```python
from build123d import *

# Parameters (mm, degrees)
SKETCH1_R           = 21
SKETCH1_R_2         = 6
BOSS_EXTRUDE1_DEPTH = 6
SKETCH2_R           = 10.5
SKETCH2_R_2         = 6
BOSS_EXTRUDE2_DEPTH = 24
SKETCH3_R           = 9.75
SKETCH3_R_2         = 6.75
CUT_EXTRUDE1_DEPTH  = 1
CUT_EXTRUDE2_START  = -7
SKETCH4_R           = 3.4
CUT_EXTRUDE2_DEPTH  = 32
CIRPATTERN1_COUNT   = 4


with BuildPart() as part:
    # Sketch1 → Boss-Extrude1 (new body)
    with BuildSketch(Plane(origin=(0, 0, 0), x_dir=(1, 0, 0), z_dir=(0, 1, 0))):
        Circle(SKETCH1_R)
        Circle(SKETCH1_R_2, mode=Mode.SUBTRACT)
    extrude(amount=BOSS_EXTRUDE1_DEPTH)

    # Sketch2 → Boss-Extrude2 (add)
    with BuildSketch(Plane(origin=(0, 6, 0), x_dir=(1, 0, 0), z_dir=(0, 1, 0))):
        Circle(SKETCH2_R)
        Circle(SKETCH2_R_2, mode=Mode.SUBTRACT)
    extrude(amount=BOSS_EXTRUDE2_DEPTH)

    # Sketch3 → Cut-Extrude1 (cut)
    with BuildSketch(Plane(origin=(0, 30, 0), x_dir=(1, 0, 0), z_dir=(0, 1, 0))):
        Circle(SKETCH3_R)
        Circle(SKETCH3_R_2, mode=Mode.SUBTRACT)
    extrude(amount=-CUT_EXTRUDE1_DEPTH, mode=Mode.SUBTRACT)

    # Sketch4 → Cut-Extrude2 (cut)
    with BuildSketch(Plane(origin=(0, 6, 0), x_dir=(1, 0, 0), z_dir=(0, 1, 0)).offset(CUT_EXTRUDE2_START)):
        with Locations((16, 0)):
            Circle(SKETCH4_R)
    cut_extrude2 = extrude(amount=CUT_EXTRUDE2_DEPTH, mode=Mode.SUBTRACT)

    # CirPattern1: Cut-Extrude2 ×4 about axis
    cirpattern1_axis = Axis((0, 0, 0), (0, 1, 0))
    for i in range(1, CIRPATTERN1_COUNT):
        add(cut_extrude2.rotate(cirpattern1_axis, i * 360 / CIRPATTERN1_COUNT), mode=Mode.SUBTRACT)


solid = part.part
```
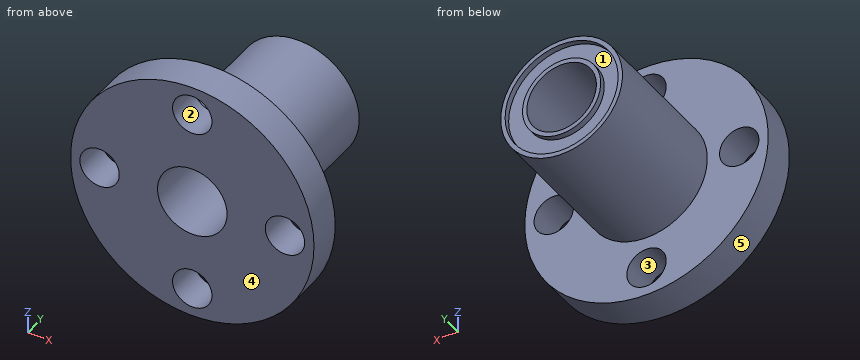
The model under review builds one solid part; all positions refer to its coordinate system, in mm. Face numbers are marked on the shaded views. A direction names the side the tool comes from. Round coordinates to 2 decimals unless told otherwise and drop trailing zeros. Loops run counter-clockwise (first coordinate to the right, second up) from the corner with the lowest first, then second, coordinate; pieces in that order, holes last.
1) Consider section C-C on z = 16. State the section outline as (x, y) points.
Values follow:
outline: (-13.6, 0) - (-3.4, 0) - (-3.4, 6) - (-13.6, 6) - close; (3.4, 0) - (13.6, 0) - (13.6, 6) - (3.4, 6) - close
2) Wall thickness on line 1 along X through (y, z) = (29.35, 0); line 2 along X through (y, z) = (18.25, 0); line 3 along Y through (x, z) = (16, -6): over which ranges is each line inside the solid? List them lowest first.
Values follow:
line 1: x = -10.5 to -9.75, -6.75 to -6, 6 to 6.75, 9.75 to 10.5
line 2: x = -10.5 to -6, 6 to 10.5
line 3: y = 0 to 6
3) Clearance check with flat-ended pins moving along their axes: P1, Ø4, axis at x = -6.5, z = 7, coming from the +Y side; P2, Ø4, axis at y = 12.5, z = 1.5, coming from the +X side; P3, Ø10, axis at x = -14, z = -16.5, coming from the +Y side; P4, Ø5, axis at x = -2.5, y = 13.5, coming from the -Z side. State where each tip first meets the part, or that it passes through.
Values follow:
P1: stops at y = 30
P2: stops at x = 10.5
P3: stops at y = 6
P4: stops at z = -10.5
4) Consider section D-D on y = 18.75. State the section outline as (x, z) points.
Values follow:
outline: circle Ø21 at (0, 0); hole circle Ø12 at (0, 0)
5) The part is to be moulded in two halves that separate along Z. For the marked faces 3, 4 and 5, say which applies: pulls with the +Z half, pulls with the -Z half, needs draft (parallel to the pull), parting line crosses it, or undercut.
Values follow:
face 3: undercut
face 4: needs draft
face 5: parting line crosses it
6) Consider section A-A on x = 0. State the section outline as (y, z) points.
Values follow:
outline: (0, -21) - (6, -21) - (6, -19.4) - (0, -19.4) - close; (0, -12.6) - (6, -12.6) - (6, -10.5) - (30, -10.5) - (30, -9.75) - (29, -9.75) - (29, -6.75) - (30, -6.75) - (30, -6) - (0, -6) - close; (0, 6) - (30, 6) - (30, 6.75) - (29, 6.75) - (29, 9.75) - (30, 9.75) - (30, 10.5) - (6, 10.5) - (6, 12.6) - (0, 12.6) - close; (0, 19.4) - (6, 19.4) - (6, 21) - (0, 21) - close
7) Tool access review of the marked faces 1 and 2: name each direction out of +Z, -Z, +X, -X, +Y, -Y from which nothing blocks a thin tool from reaching the whole face with its end or side.
Values follow:
face 1: +Y
face 2: +Y, -Y
8) Consider section B-B on z = 0. State the section outline as (x, y) points.
Values follow:
outline: (-21, 0) - (-19.4, 0) - (-19.4, 6) - (-21, 6) - close; (-12.6, 0) - (-6, 0) - (-6, 30) - (-6.75, 30) - (-6.75, 29) - (-9.75, 29) - (-9.75, 30) - (-10.5, 30) - (-10.5, 6) - (-12.6, 6) - close; (6, 0) - (12.6, 0) - (12.6, 6) - (10.5, 6) - (10.5, 30) - (9.75, 30) - (9.75, 29) - (6.75, 29) - (6.75, 30) - (6, 30) - close; (19.4, 0) - (21, 0) - (21, 6) - (19.4, 6) - close
